Design review of the part shown in the three views and the two pictorial views. Dimensions are in mm from the part's minimum x, y and z. Give positions to 0.01 mm unless a question says otherwise; leave off trailing zeros. Loops run counter-clockwise (first coordinate to the right, second up) from the corner with the lowest first, then second, coordinate; pieces in that order, holes last. Notation, with made-up numbers: (58, -8) -> (76, -8) arc R30 cw to (76, 25) -> close; hole circle Ø4 at (79.5, 17.25). An arc over 180 degrees is marked (long way). Answer as CSV lines item,"result".
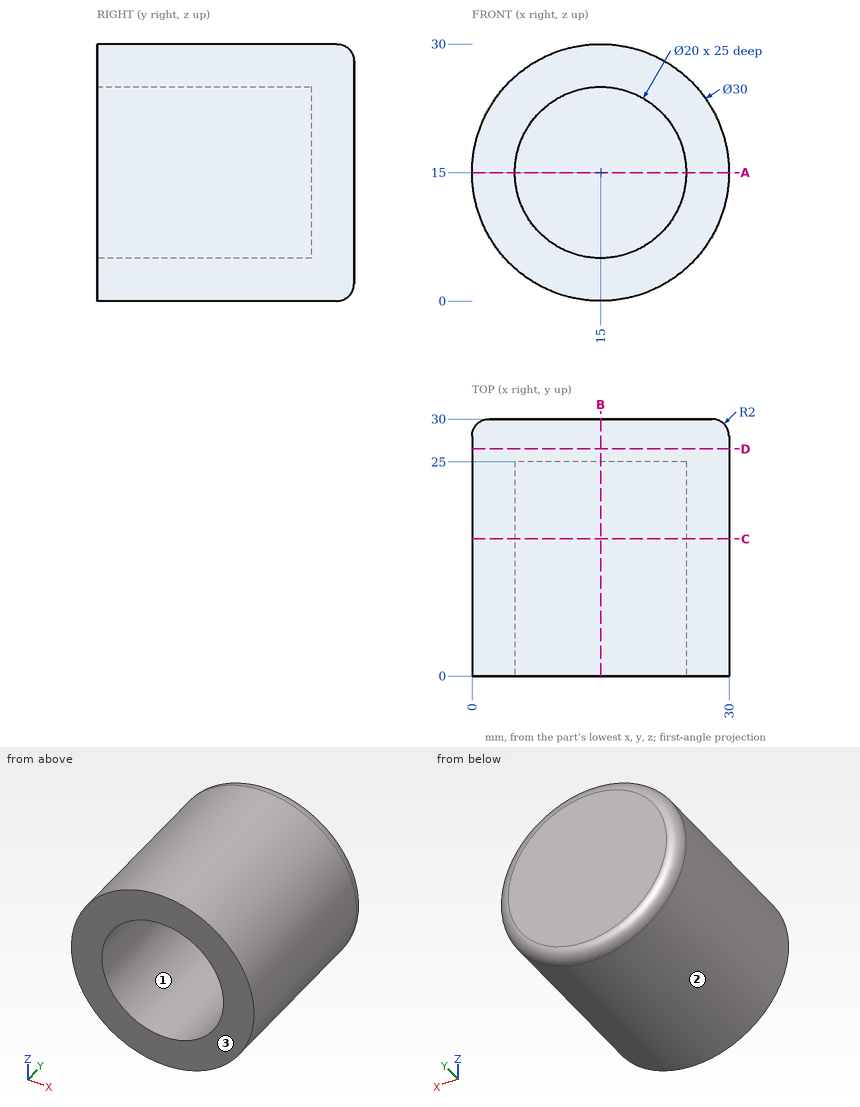
Q1. We need section B-B, the plane x = 15. State the section outline as (y, z) points.
Filled sheet:
outline,"(0, 0) -> (28, 0) arc R2 ccw to (30, 2) -> (30, 28) arc R2 ccw to (28, 30) -> (0, 30) -> (0, 25) -> (25, 25) -> (25, 5) -> (0, 5) -> close"
Q2. We need section D-D, the plane y = 26.5. State the section outline as (x, z) points, and give its area (3 significant figures).
Filled sheet:
outline,"circle Ø30 at (15, 15)"
area,"707 mm^2"
Q3. We need section C-C, the plane y = 16. State the section outline as (x, z) points, and give its area (3 significant figures).
Filled sheet:
outline,"circle Ø30 at (15, 15); hole circle Ø20 at (15, 15)"
area,"393 mm^2"
Q4. To check wall thickness, follow probe 1 along X at (y, z) = (9.75, 15); probe 2 along Y at (x, z) = (21.25, 15); probe 3 along Z at (x, y) = (24.25, 16.75). State the ranges of each line that lie inside material, in increasing order. Write a range as from..to.
Filled sheet:
probe 1,"x = 0..5, 25..30"
probe 2,"y = 25..30"
probe 3,"z = 3.19..11.2, 18.8..26.81"
Q5. We need section A-A, the plane z = 15. State the section outline as (x, y) points, and give its area (3 significant figures).
Filled sheet:
outline,"(0, 0) -> (5, 0) -> (5, 25) -> (25, 25) -> (25, 0) -> (30, 0) -> (30, 28) arc R2 ccw to (28, 30) -> (2, 30) arc R2 ccw to (0, 28) -> close"
area,"398 mm^2"
Q6. Clearance check with flat-ended pins moving along their axes: pin 1 Ø6 at (x, z) = (18.5, 13.5) entering from -Y; pin 2 Ø1 at (y, z) = (17.5, 26.5) entering from +X; pin 3 Ø1.5 at (x, y) = (13.5, 5.5) entering from +Z. State where each tip first meets the part, or that it passes through.
Filled sheet:
pin 1,"stops at y = 25"
pin 2,"stops at x = 25.2"
pin 3,"stops at z = 29.98"
Q7. The part is to be moulded in two halves that separate along Z. For the marked faces 1, 2 and 3, say which applies: pulls with the +Z half, pulls with the -Z half, needs draft (parallel to the pull), parting line crosses it, or undercut.
Filled sheet:
face 1,"undercut"
face 2,"parting line crosses it"
face 3,"needs draft"
